from build123d import *

# Parameters (mm, degrees)
SKETCH1_W           = 190.5
SKETCH1_H           = 113.82
BOSS_EXTRUDE1_DEPTH = 1.5
SKETCH2_R           = 2.2
CUT_EXTRUDE1_DEPTH  = 2.5
SKETCH3_R           = 2.2
CUT_EXTRUDE2_DEPTH  = 2.5
SKETCH4_R           = 3.25
CUT_EXTRUDE3_DEPTH  = 2.5
FILLET1_R           = 5
FILLET2_R           = 5


with BuildPart() as part:
    # Sketch1 → Boss-Extrude1 (new body)
    with BuildSketch(Plane.XY):
        with Locations((95.25, 56.91)):
            Rectangle(SKETCH1_W, SKETCH1_H)
    extrude(amount=BOSS_EXTRUDE1_DEPTH)

    # Sketch2 → Cut-Extrude1 (cut, through all)
    with BuildSketch(Plane(origin=(0, 0, 0), x_dir=(-1, 0, 0), z_dir=(0, 0, -1))):
        with Locations((-183.4, 82.41)):
            Circle(SKETCH2_R)
        with Locations((-183.4, 31.41)):
            Circle(SKETCH2_R)
        with Locations((-7.1, 31.41)):
            Circle(SKETCH2_R)
        with Locations((-7.1, 82.41)):
            Circle(SKETCH2_R)
    extrude(amount=-CUT_EXTRUDE1_DEPTH, mode=Mode.SUBTRACT)

    # Sketch3 → Cut-Extrude2 (cut, through all)
    with BuildSketch(Plane(origin=(0, 0, 0), x_dir=(-1, 0, 0), z_dir=(0, 0, -1))):
        with Locations((-95.25, 107.31)):
            Circle(SKETCH3_R)
        with Locations((-39.45, 107.31)):
            Circle(SKETCH3_R)
        with Locations((-151.05, 107.31)):
            Circle(SKETCH3_R)
        with Locations((-39.45, 6.51)):
            Circle(SKETCH3_R)
        with Locations((-95.25, 6.51)):
            Circle(SKETCH3_R)
        with Locations((-151.05, 6.51)):
            Circle(SKETCH3_R)
    extrude(amount=-CUT_EXTRUDE2_DEPTH, mode=Mode.SUBTRACT)

    # Sketch4 → Cut-Extrude3 (cut, through all)
    with BuildSketch(Plane(origin=(0, 0, 0), x_dir=(-1, 0, 0), z_dir=(0, 0, -1))):
        with Locations((-151.05, 56.91)):
            Circle(SKETCH4_R)
        with Locations((-123.05, 56.91)):
            Circle(SKETCH4_R)
        with Locations((-95.05, 56.91)):
            Circle(SKETCH4_R)
        with Locations((-67.05, 56.91)):
            Circle(SKETCH4_R)
        with BuildLine():
            Line((-153.499489743, 89.71), (-148.600510257, 89.71))
            ThreePointArc((-148.600510257, 89.71), (-143.35, 82.41), (-148.600510257, 75.11))
            Line((-148.600510257, 75.11), (-153.499489743, 75.11))
            ThreePointArc((-153.499489743, 75.11), (-158.75, 82.41), (-153.499489743, 89.71))
        make_face()
        with BuildLine():
            Line((-153.499489743, 24.11), (-148.600510257, 24.11))
            ThreePointArc((-148.600510257, 24.11), (-143.35, 31.41), (-148.600510257, 38.71))
            Line((-148.600510257, 38.71), (-153.499489743, 38.71))
            ThreePointArc((-153.499489743, 38.71), (-158.75, 31.41), (-153.499489743, 24.11))
        make_face()
        with BuildLine():
            Line((-125.499489743, 75.11), (-120.600510257, 75.11))
            ThreePointArc((-120.600510257, 75.11), (-115.35, 82.41), (-120.600510257, 89.71))
            Line((-120.600510257, 89.71), (-125.499489743, 89.71))
            ThreePointArc((-125.499489743, 89.71), (-130.75, 82.41), (-125.499489743, 75.11))
        make_face()
        with BuildLine():
            Line((-125.499489743, 38.71), (-120.600510257, 38.71))
            ThreePointArc((-120.600510257, 38.71), (-115.35, 31.41), (-120.600510257, 24.11))
            Line((-120.600510257, 24.11), (-125.499489743, 24.11))
            ThreePointArc((-125.499489743, 24.11), (-130.75, 31.41), (-125.499489743, 38.71))
        make_face()
        with BuildLine():
            Line((-97.499489743, 75.11), (-92.600510257, 75.11))
            ThreePointArc((-92.600510257, 75.11), (-87.35, 82.41), (-92.600510257, 89.71))
            Line((-92.600510257, 89.71), (-97.499489743, 89.71))
            ThreePointArc((-97.499489743, 89.71), (-102.75, 82.41), (-97.499489743, 75.11))
        make_face()
        with BuildLine():
            Line((-97.499489743, 38.71), (-92.600510257, 38.71))
            ThreePointArc((-92.600510257, 38.71), (-87.35, 31.41), (-92.600510257, 24.11))
            Line((-92.600510257, 24.11), (-97.499489743, 24.11))
            ThreePointArc((-97.499489743, 24.11), (-102.75, 31.41), (-97.499489743, 38.71))
        make_face()
        with BuildLine():
            Line((-69.499489743, 75.11), (-64.600510257, 75.11))
            ThreePointArc((-64.600510257, 75.11), (-59.35, 82.41), (-64.600510257, 89.71))
            Line((-64.600510257, 89.71), (-69.499489743, 89.71))
            ThreePointArc((-69.499489743, 89.71), (-74.75, 82.41), (-69.499489743, 75.11))
        make_face()
        with BuildLine():
            Line((-69.499489743, 38.71), (-64.600510257, 38.71))
            ThreePointArc((-64.600510257, 38.71), (-59.35, 31.41), (-64.600510257, 24.11))
            Line((-64.600510257, 24.11), (-69.499489743, 24.11))
            ThreePointArc((-69.499489743, 24.11), (-74.75, 31.41), (-69.499489743, 38.71))
        make_face()
        with BuildLine():
            Line((-41.499489743, 75.11), (-36.600510257, 75.11))
            ThreePointArc((-36.600510257, 75.11), (-31.35, 82.41), (-36.600510257, 89.71))
            Line((-36.600510257, 89.71), (-41.499489743, 89.71))
            ThreePointArc((-41.499489743, 89.71), (-46.75, 82.41), (-41.499489743, 75.11))
        make_face()
        with BuildLine():
            Line((-41.499489743, 38.71), (-36.600510257, 38.71))
            ThreePointArc((-36.600510257, 38.71), (-31.35, 31.41), (-36.600510257, 24.11))
            Line((-36.600510257, 24.11), (-41.499489743, 24.11))
            ThreePointArc((-41.499489743, 24.11), (-46.75, 31.41), (-41.499489743, 38.71))
        make_face()
    extrude(amount=-CUT_EXTRUDE3_DEPTH, mode=Mode.SUBTRACT)

    # Fillet1
    fillet1_edges = [part.edges().sort_by_distance(p)[0] for p in [
        (190.5, 113.82, 0.75),
        (190.5, 0, 0.75),
    ]]
    fillet(fillet1_edges, radius=FILLET1_R)

    # Fillet2
    fillet2_edges = [part.edges().sort_by_distance(p)[0] for p in [
        (0, 113.82, 0.75),
        (0, 0, 0.75),
    ]]
    fillet(fillet2_edges, radius=FILLET2_R)


solid = part.part
Geometry check sheet. Reference: the model listing, model coordinates, mm. A direction names the side the tool comes from. Give positions to 0.01 mm unless a question says otherwise; leave off trailing zeros. Write each loop counter-clockwise with the first axis right and the second up, starting at its lowest first coordinate (ties: lowest second). Pieces come first, ordered by that corner, then holes. Notation, with made-up numbers: M -13.5,58 L 22.5,58 A18 cw 22.5,80 Z; hole C 47,-32 d7. An arc over 180 degrees is marked long. Answer as CSV lines item,"result". Start each with the question number.
Q1. Section check B-B, the plane x = 39.45. Record the cut outline in (y, z).
Q2. Section check C-C, the plane x = 151.05. Record the cut outline in (y, z), then the cut area to 3 significant figures.
Q3. Material ranges on L1, parallel to Y at x = 67.05, z = 1.1; L2, parallel to Y at x = 67.5, z = 1.35; L3, parallel to Y at x = 95.25, z = 0.45, recorded low to high.
Q4. Tool access check on faces 1 (the face through (94, 70, 1.5)), 2 (the face through (102.75, 82.54, 0.74)). Record the directions out of +Z, -Z, +X, -X, +Y, -Y that give a thin tool (end or side, any length) a straight path to the whole face; none if there is none.
Q5. Section check D-D, the plane x = 123.05. Record the cut outline in (y, z), then the cut area to 3 significant figures.
Q6. Section check A-A, the plane y = 56.91. Record the cut outline in (x, z).
Q7. Release check for a two-part mould opening along X. For faces 3 (the face through (94, 70, 0)), 4 (the face through (189, 112.39, 0.76)), 5 (the face through (59.35, 31.54, 0.74)), 6 (the face through (7.39, 33.59, 0.74)) record: pulls with the +X half, pulls with the -X half, needs draft (parallel to the pull), parting line crosses it, or undercut.
Geometry says:
1,outline,"M 0,0 L 4.31,0 L 4.31,1.5 L 0,1.5 Z; M 8.71,0 L 24.11,0 L 24.11,1.5 L 8.71,1.5 Z; M 38.71,0 L 75.11,0 L 75.11,1.5 L 38.71,1.5 Z; M 89.71,0 L 105.11,0 L 105.11,1.5 L 89.71,1.5 Z; M 109.51,0 L 113.82,0 L 113.82,1.5 L 109.51,1.5 Z"
2,outline,"M 0,0 L 4.31,0 L 4.31,1.5 L 0,1.5 Z; M 8.71,0 L 24.11,0 L 24.11,1.5 L 8.71,1.5 Z; M 38.71,0 L 53.66,0 L 53.66,1.5 L 38.71,1.5 Z; M 60.16,0 L 75.11,0 L 75.11,1.5 L 60.16,1.5 Z; M 89.71,0 L 105.11,0 L 105.11,1.5 L 89.71,1.5 Z; M 109.51,0 L 113.82,0 L 113.82,1.5 L 109.51,1.5 Z"
2,area,"104 mm^2"
3,L1,"0 to 24.11, 38.71 to 53.66, 60.16 to 75.11, 89.71 to 113.82"
3,L2,"0 to 24.11, 38.71 to 53.69, 60.13 to 75.11, 89.71 to 113.82"
3,L3,"0 to 4.31, 8.71 to 24.11, 38.71 to 53.67, 60.15 to 75.11, 89.71 to 105.11, 109.51 to 113.82"
4,face 1,"+Z, +X, -X, +Y, -Y"
4,face 2,"+Z, -Z"
5,outline,"M 0,0 L 24.11,0 L 24.11,1.5 L 0,1.5 Z; M 38.71,0 L 53.66,0 L 53.66,1.5 L 38.71,1.5 Z; M 60.16,0 L 75.11,0 L 75.11,1.5 L 60.16,1.5 Z; M 89.71,0 L 113.82,0 L 113.82,1.5 L 89.71,1.5 Z"
5,area,"117 mm^2"
6,outline,"M 0,0 L 63.8,0 L 63.8,1.5 L 0,1.5 Z; M 70.3,0 L 91.8,0 L 91.8,1.5 L 70.3,1.5 Z; M 98.3,0 L 119.8,0 L 119.8,1.5 L 98.3,1.5 Z; M 126.3,0 L 147.8,0 L 147.8,1.5 L 126.3,1.5 Z; M 154.3,0 L 190.5,0 L 190.5,1.5 L 154.3,1.5 Z"
7,face 3,"needs draft"
7,face 4,"pulls with the +X half"
7,face 5,"undercut"
7,face 6,"undercut"
